Part model, mm, in its own coordinate system. A direction names the side the tool comes from. Round coordinates to 2 decimals unless told otherwise and drop trailing zeros. Loops run counter-clockwise (first coordinate to the right, second up) from the corner with the lowest first, then second, coordinate; pieces in that order, holes last.
(1) Cut at A-A on z = 33.5. List the corners of the cut face in (x, y).
(2) Flat gauge pins, fed straight in: pin 1 (1.5 mm diameter, centred on x = -27.5, y = 27, fed in from -Z); pin 2 (3.5 mm diameter, centred on x = -27.21, y = 27.24, fed in from +Z); pin 3 (12 mm diameter, centred on y = 10, z = -4.5, fed in from +X); pin 4 (12 mm diameter, centred on x = 29.5, z = 6.5, fed in from +Y). Where does each tip first touch, or does it go through?
(3) Mould opens along Z. For faces 5 (the face through (7.3, 7.3, -52)), 6 (the face through (27.114, -24.988, -49.493)), 7 (the face through (-29.11, 26.7, -20.49)) say: +Z half, -Z half, draft (parallel to the pull), parting line (faces both ways), or undercut.
(4) Probe probe 1 along X at (y, z) = (1, -43); probe 2 along Z at (x, y) = (-23, -5.5); probe 3 along X at (y, z) = (12, -32.5). List the from-to ranges inside material, lowest first.
(5) Tool access for faces 1 (the face through (13, 36, -50)), 2 (the face through (-36, 13, -50)), 3 (the face through (14.717, -37.076, -49.493)), 4 (the face through (-13, -36, -50)): list every direction of +Z, -Z, +X, -X, +Y, -Y with a clear straight run to the whole face (end or side of a thin tool).
Autodesk Fusion 360 part; units mm, degrees
sketch "Sketch1" plane through (0, 0, 0) normal (0, 1, 0) x (1, 0, 0)
  line L0 (0, 0) -> (-35, 0)
  line L1 (0, 0) -> (0, 20)
  line L2 (0, 20) -> (-42, 20)
  arc A0 (-42, 20) -> (-35, 0) centre (-17.1273, 17.4804) ccw
  dimension "d1" = 35
  dimension "d2" = 20
  dimension "d3" = 42
  dimension "d4" = 25
revolve "Revolve1" add sketch "Sketch1" angle 360 about axis through (0, 0, 0) along (0, 0, -1) in component "Component"
sketch "Sketch2" plane through (0, 0, -20) normal (0, 0, -1) x (1, 0, 0)
  circle A0 centre (0, 0) radius 42
  circle A1 centre (0, 0) radius 39.5
  dimension "d6" = 79
extrude "Extrude1" add sketch "Sketch2" along normal blind 1 contours A1 in component "Component"
sketch "Sketch3" plane through (0, 0, 0) normal (1, 0, 0) x (0, 1, 0)
  line L0 (0, -21) -> (0, -41)
  line L1 (0, -41) -> (-42, -41)
  line L2 (0, -21) -> (-40, -21)
  arc A0 (-40, -21) -> (-42, -41) centre (-5.5677, -34.5432) ccw
  dimension "d9" = 20
  dimension "d10" = 42
  dimension "d11" = 40
  dimension "d12" = 37
revolve "Revolve2" add sketch "Sketch3" angle 360 about axis through (0, 0, -21) along (0, 0, -1) in component "Component"
sketch "Sketch4" plane through (0, 0, -41) normal (0, 0, -1) x (1, 0, 0)
  circle A0 centre (0, 0) radius 42
  circle A1 centre (0, 0) radius 41
  dimension "d14" = 82
extrude "Extrude2" add sketch "Sketch4" along normal blind 1 contours A1 in component "Component"
sketch "Sketch5" plane through (0, 0, -42) normal (0, 0, -1) x (1, 0, 0)
  circle A0 centre (0, 0) radius 41
  circle A1 centre (0, 0) radius 42
  dimension "d17" = 84
extrude "Extrude3" add sketch "Sketch5" along normal blind 7 contours A0 | A1 in component "Component"
sketch "Sketch6" plane through (0, 0, -49) normal (0, 0, -1) x (1, 0, 0)
  circle A0 centre (0, 0) radius 42
  circle A1 centre (0, 0) radius 35
  dimension "d20" = 70
extrude "Extrude4" add sketch "Sketch6" along normal blind 3 contours A1 in component "Component"
sketch "Sketch7" plane through (0, 0, -49) normal (0, 0, -1) x (1, 0, 0)
  circle A0 centre (0, 0) radius 35
  circle A1 centre (0, 0) radius 42
  line L0 (35, 0.0167) -> (42, 0.0167)
  circle A2 centre (38.5, 0.0167) radius 2.25
  circle A3 centre (38.5, 0.0167) radius 1.5
  dimension "d23" = 4.5
  dimension "d24" = 3
extrude "Extrude5" add sketch "Sketch7" along normal blind 1 contours L0 A2 A3 | L0 A2 A3 in component "Component"
pattern_circular "C-Pattern1" count 16 over 360 about axis through (0, 0, -49) along (0, 0, 1) of "Extrude5" in component "Component"
sketch "Sketch8" plane through (0, 0, 0) normal (0, 0, 1) x (-1, 0, 0)
  circle A0 centre (0, 0) radius 35
  line L0 (12, 20) -> (-12, 20)
  line L1 (-12, 20) -> (-12, -20)
  line L2 (-12, -20) -> (12, -20)
  line L3 (12, -20) -> (12, 20)
  line L4 (12, 20) -> (-12, -20) construction
  line L5 (-12, 20) -> (12, -20) construction
  dimension "d29" = 24
  dimension "d30" = 40
extrude "Extrude6" add sketch "Sketch8" along normal blind 42 contours L0 L1 L2 L3 in component "Component"
sketch "Sketch9" plane through (12, 0, 0) normal (1, 0, 0) x (0, 1, 0)
  line L0 (-20, 0) -> (20, 0)
  line L1 (20, 0) -> (20, 42)
  line L2 (20, 42) -> (-20, 42)
  line L3 (-20, 42) -> (-20, 0)
  circle A0 centre (0, 42) radius 20
extrude "Extrude7" add sketch "Sketch9" against normal blind 24 contours L2 A0 picked at (4.1566, 47.2122) in component "Component"
sketch "Sketch10" plane through (12, 0, 0) normal (1, 0, 0) x (0, 1, 0)
  line L0 (-20, 0) -> (20, 0)
  line L1 (20, 0) -> (20, 42)
  arc A0 (20, 42) -> (-20, 42) centre (0, 42) ccw
  line L2 (-20, 42) -> (-20, 0)
  circle A1 centre (0, 42) radius 10
  dimension "d35" = 20
extrude "Extrude8" add sketch "Sketch10" along normal blind 10 contours A1 in component "Component"
sketch "Sketch11" plane through (0, 0, -52) normal (0, 0, -1) x (1, 0, 0)
  circle A0 centre (0, 0) radius 35
  circle A1 centre (0, 0) radius 10
  dimension "d38" = 20
extrude "Extrude9" add sketch "Sketch11" along normal blind 10 contours A1 in component "Component"
component "Component" placed x (1, 0, 0) y (0, 1, 0) z (0, 0, 1) at (0, 0, 0)
Final values:
1. outline: (-12, -20) - (12, -20) - (12, -5.27) - (22, -5.27) - (22, 5.27) - (12, 5.27) - (12, 20) - (-12, 20) - close
2. pin 1: stops at z = -49
2. pin 2: stops at z = -1.99
2. pin 3: stops at x = 40.28
2. pin 4: passes through
3. face 5: -Z half
3. face 6: draft
3. face 7: undercut
4. probe 1: x = -41.99 to 41.99
4. probe 2: z = -52 to 0
4. probe 3: x = -40.78 to 40.78
5. face 1: -Z, +X, +Y
5. face 2: -Z, -X, +Y
5. face 3: -Z
5. face 4: -Z, -X, -Y
